```python
from build123d import *

# Parameters (mm, degrees)
SKETCH_R        = 1.5
PAD_DEPTH       = 2
FILLET001_R     = 5
SKETCH003_W     = 42
SKETCH003_H     = 23
POCKET001_DEPTH = 1.5
SKETCH004_W     = 42
SKETCH004_H     = 5
SKETCH004_R     = 1.5
PAD002_DEPTH    = 5
FILLET002_R     = 4
SKETCH007_W     = 1
SKETCH007_H     = 20
SKETCH007_W_2   = 2
SKETCH007_H_2   = 23
PAD004_DEPTH    = 1


with BuildPart() as part:
    # Sketch → Pad (new body)
    with BuildSketch(Plane.XY):
        Polygon((-47, 20), (47, 20), (47, -20), (-47, -20), (-47, -10), (-39.75, -10), (-39.75, 10), (-47, 10), align=None)
        with Locations((-42.85, 15)):
            Circle(SKETCH_R, mode=Mode.SUBTRACT)
        with Locations((-42.85, -15)):
            Circle(SKETCH_R, mode=Mode.SUBTRACT)
        with Locations((42.85, -15)):
            Circle(SKETCH_R, mode=Mode.SUBTRACT)
        with Locations((42.85, 15)):
            Circle(SKETCH_R, mode=Mode.SUBTRACT)
    extrude(amount=PAD_DEPTH)

    # Fillet001
    fillet001_edges = [part.edges().sort_by_distance(p)[0] for p in [
        (47, -20, 1),
        (47, 20, 1),
        (-47, -20, 1),
        (-47, 20, 1),
    ]]
    fillet(fillet001_edges, radius=FILLET001_R)

    # Sketch003 (on Face2 of Fillet001) → Pocket001 (cut)
    with BuildSketch(Plane(origin=(0, 0, 0), x_dir=(1, 0, 0), z_dir=(0, 0, -1))):
        with Locations((-17.75, 0.5)):
            Rectangle(SKETCH003_W, SKETCH003_H)
    extrude(amount=-POCKET001_DEPTH, mode=Mode.SUBTRACT)

    # Sketch004 (on Face2 of Pocket001) → Pad002 (join)
    with BuildSketch(Plane(origin=(0, 0, 0), x_dir=(1, 0, 0), z_dir=(0, 0, -1))):
        with Locations((-17.75, 14.5)):
            Rectangle(SKETCH004_W, SKETCH004_H)
        with Locations((-26.25, 14.5)):
            Circle(SKETCH004_R, mode=Mode.SUBTRACT)
        with Locations((-9.25, 14.5)):
            Circle(SKETCH004_R, mode=Mode.SUBTRACT)
        with Locations((-17.75, -13.5)):
            Rectangle(SKETCH004_W, SKETCH004_H)
        with Locations((-26.25, -13.5)):
            Circle(SKETCH004_R, mode=Mode.SUBTRACT)
        with Locations((-9.25, -13.5)):
            Circle(SKETCH004_R, mode=Mode.SUBTRACT)
    extrude(amount=PAD002_DEPTH)

    # Fillet002
    fillet002_edges = [part.edges().sort_by_distance(p)[0] for p in [
        (3.25, 16, -2.5),
        (3.25, -17, -2.5),
        (-38.75, 16, -2.5),
        (-38.75, -17, -2.5),
    ]]
    fillet(fillet002_edges, radius=FILLET002_R)

    # Sketch007 (on Face1 of Fillet002) → Pad004 (join)
    with BuildSketch(Plane(origin=(0, 0, 0), x_dir=(1, 0, 0), z_dir=(0, 0, -1))):
        with Locations((-39.25, 0)):
            Rectangle(SKETCH007_W, SKETCH007_H)
        with Locations((4.25, 0.5)):
            Rectangle(SKETCH007_W_2, SKETCH007_H_2)
    extrude(amount=PAD004_DEPTH)


with BuildPart() as part_1:
    # Body placement: moved
    add(part.part.moved(Location((77, -1, 17))))


solid = part_1.part
```
The listing builds one solid part. Answer for the finished solid, in the listing's coordinates (mm). A direction names the side the tool comes from. Give positions to 0.01 mm unless a question says otherwise; leave off trailing zeros. Loops run counter-clockwise (first coordinate to the right, second up) from the corner with the lowest first, then second, coordinate; pieces in that order, holes last. Notation, with made-up numbers: (47.25, -34) - (52.25, -34) arc R35 ccw to (52.25, 4) - close; hole circle Ø10 at (-26.75, -38). An arc over 180 degrees is marked (long way). Return JSON: item names as keys, results as strings. Group by question number.
1. Find section A-A (z = 15). Write down the section's boundary in (x, y).
2. Determine the mould class of faces 5 (the flat face through (34, 9, 18)), 6 (the cylindrical face through (121.28, 14.45, 17.99)), 7 (the cylindrical face through (123, -19, 18)), 8 (the flat face through (30, -14, 18)) for opening direction Y: pulls with the +Y half, pulls with the -Y half, needs draft (parallel to the pull), parting line crosses it, or undercut.
3. Find section D-D (x = 67.75). Write down the section's boundary in (y, z).
4. Which of the six approach directions +Z, -Z, +X, -X, +Y, -Y give full straight-line access (tool end or side, diameter ignored) to faces 1 (the flat face through (59, 15, 15)), 2 (the cylindrical face through (79.047, 13.859, 14.465)), 3 (the cylindrical face through (39.391, 13.797, 14.465)), 4 (the flat face through (59, -13, 15))?
5. Find section B-B (x = 34.15). Write down the section's boundary in (y, z), then the cut area to 3 significant figures.
6. Find section C-C (y = -5). Write down the section's boundary in (x, z), then the cut area to 4 significant figures.
7. Straight lines are drawn through the part: line 1 (Y direction, x = 63, z = 16.5); line 2 (X direction, y = -15.5, z = 13.1); line 3 (X direction, y = -16.5, z = 15.5). For each, find the intervals that lie inside material, in ascending order. Write a range as [from, to].
8. Given pin 1 Ø10 at (x, y) = (112.5, 1.5) entering from -Z; pin 2 Ø2 at (y, z) = (-5, 17.5) entering from -X; pin 3 Ø10 at (x, y) = (78.5, -0.5) entering from -Z, each flat-ended and moving along its own axis, determine where each tip first touches the part or whether it passes through.
Verdict:
{
 "1": {"outline": "(38.25, -14) arc R4 ccw to (42.25, -18) - (76.25, -18) arc R4 ccw to (80.25, -14) - (80.25, -13) - (38.25, -13) - close; (38.25, 10) - (80.25, 10) - (80.25, 11) arc R4 ccw to (76.25, 15) - (42.25, 15) arc R4 ccw to (38.25, 11) - close; hole circle Ø3 at (50.75, -15.5); hole circle Ø3 at (50.75, 12.5); hole circle Ø3 at (67.75, -15.5); hole circle Ø3 at (67.75, 12.5)"},
 "2": {"face 5": "undercut", "face 6": "undercut", "face 7": "pulls with the -Y half", "face 8": "needs draft"},
 "3": {"outline": "(-21, 17) - (-18, 17) - (-18, 12) - (-17, 12) - (-17, 17) - (-14, 17) - (-14, 12) - (-13, 12) - (-13, 18.5) - (10, 18.5) - (10, 12) - (11, 12) - (11, 17) - (14, 17) - (14, 12) - (15, 12) - (15, 17) - (19, 17) - (19, 19) - (-21, 19) - close"},
 "4": {"face 1": "-Z, +X, -X, +Y", "face 2": "-Z, +X, +Y", "face 3": "-Z, -X, +Y", "face 4": "-Z"},
 "5": {"outline": "(-20.93, 17) - (-17.5, 17) - (-17.5, 19) - (-20.93, 19) - close; (-14.5, 17) - (-11, 17) - (-11, 19) - (-14.5, 19) - close; (9, 17) - (12.5, 17) - (12.5, 19) - (9, 19) - close; (15.5, 17) - (18.93, 17) - (18.93, 19) - (15.5, 19) - close", "area": "27.7 mm^2"},
 "6": {"outline": "(37.25, 16) - (38.25, 16) - (38.25, 18.5) - (80.25, 18.5) - (80.25, 16) - (82.25, 16) - (82.25, 17) - (124, 17) - (124, 19) - (37.25, 19) - close", "area": "113.5 mm^2"},
 "7": {"line 1": "y = [-18, -13], [10, 15]", "line 2": "x = [38.54, 49.25], [52.25, 66.25], [69.25, 79.96]", "line 3": "x = [39.13, 49.63], [51.87, 66.63], [68.87, 79.37]"},
 "8": {"pin 1": "stops at z = 17", "pin 2": "stops at x = 37.25", "pin 3": "stops at z = 16"}
}
